```python
from build123d import *

# Parameters (mm, degrees)
SKETCH1_R           = 9
SKETCH1_R_2         = 1.2
BOSS_EXTRUDE1_DEPTH = 3
BOSS_EXTRUDE2_DEPTH = 20
CHAMFER1_SIZE       = 1
SKETCH4_R           = 1.7
CUT_EXTRUDE1_DEPTH  = 29.487378672
SKETCH5_R           = 1.7
CUT_EXTRUDE2_DEPTH  = 29.896366633


with BuildPart() as part:
    # Sketch1 → Boss-Extrude1 (new body)
    with BuildSketch(Plane(origin=(0, 0, 0), x_dir=(0, 0, -1), z_dir=(1, 0, 0))):
        Circle(SKETCH1_R)
        with Locations((0, 6)):
            Circle(SKETCH1_R_2, mode=Mode.SUBTRACT)
        with Locations((6, 0)):
            Circle(SKETCH1_R_2, mode=Mode.SUBTRACT)
        with Locations((-6, 0)):
            Circle(SKETCH1_R_2, mode=Mode.SUBTRACT)
        with Locations((0, -6)):
            Circle(SKETCH1_R_2, mode=Mode.SUBTRACT)
    extrude(amount=BOSS_EXTRUDE1_DEPTH)

    # Sketch2 → Boss-Extrude2 (add)
    with BuildSketch(Plane(origin=(3, 0, 0), x_dir=(0, 0, -1), z_dir=(1, 0, 0))):
        with BuildLine():
            Line((2.367240814, -5.196152423), (3, -5.196152423))
            Line((3, -5.196152423), (4.75, -2.165063509))
            ThreePointArc((4.75, -2.165063509), (3.5, 0), (4.75, 2.165063509))
            Line((4.75, 2.165063509), (3, 5.196152423))
            Line((3, 5.196152423), (2.367240814, 5.196152423))
            ThreePointArc((2.367240814, 5.196152423), (0, 3.5), (-2.367240814, 5.196152423))
            Line((-2.367240814, 5.196152423), (-3, 5.196152423))
            Line((-3, 5.196152423), (-4.75, 2.165063509))
            ThreePointArc((-4.75, 2.165063509), (-3.5, 0), (-4.75, -2.165063509))
            Line((-4.75, -2.165063509), (-3, -5.196152423))
            Line((-3, -5.196152423), (-2.367240814, -5.196152423))
            ThreePointArc((-2.367240814, -5.196152423), (0, -3.5), (2.367240814, -5.196152423))
        make_face()
    extrude(amount=BOSS_EXTRUDE2_DEPTH)

    # Chamfer1
    chamfer1_edges = [part.edges().sort_by_distance(p)[0] for p in [
        (3, -3.680607966, 3.875),
        (3, -5.196152423, 2.683620407),
        (3, -5.196152423, -2.683620407),
        (3, -3.680607966, -3.875),
        (3, 3.680607966, -3.875),
        (3, 5.196152423, -2.683620407),
        (3, 5.196152423, 2.683620407),
        (3, 3.680607966, 3.875),
    ]]
    chamfer(chamfer1_edges, length=CHAMFER1_SIZE)

    # Sketch4 → Cut-Extrude1 (cut, through all)
    with BuildSketch(Plane.XZ.offset(5.196152423)):
        with Locations(Location((13, 0, 0), (0, 0, 270))):
            Circle(SKETCH4_R)
    extrude(amount=-CUT_EXTRUDE1_DEPTH, mode=Mode.SUBTRACT)

    # Sketch5 → Cut-Extrude2 (cut, through all)
    with BuildSketch(Plane.XY.offset(6)):
        with Locations((13, 0)):
            Circle(SKETCH5_R)
    extrude(amount=-CUT_EXTRUDE2_DEPTH, mode=Mode.SUBTRACT)


solid = part.part
```
Input: part model. Units: mm. Frame: model coordinates. A direction names the side the tool comes from. Give positions to 0.01 mm unless a question says otherwise; leave off trailing zeros. Order: outer loops, then holes, each group sorted by start corner. A loop starts at its lowest first (then second) coordinate and runs counter-clockwise, first axis right, second up. Notation, with made-up numbers: (84.5, 69.5) -> (118.5, 69.5) arc R25 ccw to (118.5, 100.5) -> close; hole circle Ø10 at (28.25, 66). An arc over 180 degrees is marked (long way). Write each question's results on one line, items separated by ' | '. Start each with the question number.
Item 1: Cut plane B-B on y = 0.5. Return the cut outline in (x, z), then the cut area to 3 significant figures.
Item 2: Contact query for flat-ended pins moving along their axis: P1, Ø6, axis at x = 7.5, y = 4, coming from the +Z side; P2, Ø6, axis at x = 17, y = 7, coming from the +Z side; P3, Ø0.5, axis at x = 13.5, z = 3, coming from the +Y side. Output: stop coordinate, or through.
Item 3: Set-up query: faces 5 (the cylindrical face through (12.9, -2, 4.5)), 6 (the flat face through (13.367, 3.659, -3.887)), 7 (the flat face through (13.367, -3.659, 3.887)), 8 (the flat face through (13.367, -3.702, -3.863)). Return all of +Z, -Z, +X, -X, +Y, -Y with unobstructed straight access to the full face (end or side cutting, diameter ignored); none if empty.
Item 4: Mould query, pull axis Z, two halves, no side actions, for faces 1 (the flat face through (3.51, 4.11, 4.19)), 2 (the cylindrical face through (12.9, 2, -4.5)), 3 (the cylindrical face through (13.51, -2.58, -1.62)), 4 (the cylindrical face through (1.48, 0.05, 7.2)). Classes: pulls with the +Z half, pulls with the -Z half, needs draft (parallel to the pull), parting line crosses it, or undercut.
Item 5: Cut plane C-C on z = 6. Return the cut outline in (x, y).
Item 6: Cut plane A-A on x = 13. Return the cut outline in (y, z).
Item 7: Line query: line 1 (Y direction, x = 2.05, z = 0); line 2 (X direction, y = -3.3, z = 0); line 3 (Y direction, x = 7.25, z = 2.75). Output: solid intervals per line, ascending.
Item 8: Cut plane D-D on x = 15.5. Return the cut outline in (y, z), then the cut area to 3 significant figures.
Established:
1) outline: (0, -8.99) -> (3, -8.99) -> (3, -7.09) -> (0, -7.09) -> close; (0, -4.91) -> (3, -4.91) -> (3, -3.55) -> (11.38, -3.55) -> (11.38, -0.5) arc R1.7 cw to (11.38, 0.5) -> (11.38, 3.55) -> (3, 3.55) -> (3, 4.91) -> (0, 4.91) -> close; (0, 7.09) -> (3, 7.09) -> (3, 8.99) -> (0, 8.99) -> close; (14.62, -3.55) -> (23, -3.55) -> (23, 3.55) -> (14.62, 3.55) -> (14.62, 0.5) arc R1.7 cw to (14.62, -0.5) -> close | area: 160 mm^2
2) P1: z = 4.75 | P2: z = 3.69 | P3: y = 5.2
3) face 5: +Z, +X | face 6: -Z, +X, +Y | face 7: +Z, +X, -Y | face 8: -Z, +X, -Y
4) face 1: pulls with the +Z half | face 2: pulls with the -Z half | face 3: undercut | face 4: undercut
5) outline: (0, -6.71) -> (3, -6.71) -> (3, -1.2) -> (0, -1.2) -> close; (0, 1.2) -> (3, 1.2) -> (3, 6.71) -> (0, 6.71) -> close
6) outline: (-5.2, -3) -> (-2.17, -4.75) arc R2.5 cw to (-1.7, -4.17) -> (-1.7, -1.7) -> (-4.17, -1.7) arc R2.5 cw to (-5.2, -2.37) -> close; (-5.2, 2.37) arc R2.5 cw to (-4.17, 1.7) -> (-1.7, 1.7) -> (-1.7, 4.17) arc R2.5 cw to (-2.17, 4.75) -> (-5.2, 3) -> close; (1.7, -4.17) arc R2.5 cw to (2.17, -4.75) -> (5.2, -3) -> (5.2, -2.37) arc R2.5 cw to (4.17, -1.7) -> (1.7, -1.7) -> close; (1.7, 1.7) -> (4.17, 1.7) arc R2.5 cw to (5.2, 2.37) -> (5.2, 3) -> (2.17, 4.75) arc R2.5 cw to (1.7, 4.17) -> close
7) line 1: -9 to -7.2, -4.8 to 4.8, 7.2 to 9 | line 2: 0 to 11.3, 14.7 to 23 | line 3: -5.2 to 5.2
8) outline: (-5.2, -3) -> (-2.17, -4.75) arc R2.5 cw to (2.17, -4.75) -> (5.2, -3) -> (5.2, -2.37) arc R2.5 cw to (5.2, 2.37) -> (5.2, 3) -> (2.17, 4.75) arc R2.5 cw to (-2.17, 4.75) -> (-5.2, 3) -> (-5.2, 2.37) arc R2.5 cw to (-5.2, -2.37) -> close | area: 68.7 mm^2
